Build history of the part. All positions in model axes, mm. A direction names the side the tool comes from. Give positions to 0.01 mm unless a question says otherwise; leave off trailing zeros. Write each loop counter-clockwise with the first axis right and the second up, starting at its lowest first coordinate (ties: lowest second). Pieces come first, ordered by that corner, then holes. Notation, with made-up numbers: (76.25, -11) -> (112.25, -11) arc R19 cw to (112.25, 0) -> close; hole circle Ø6 at (18, 19). An arc over 180 degrees is marked (long way). Write item = value, one per line. Start each with the question number.
Q1. Mould opens along X. For faces 1 (the face through (0, 28, 0)), 2 (the face through (-56, 1, 0)), 3 (the face through (-1, 1, 13.5)) say: pulls with the +X half, pulls with the -X half, needs draft (parallel to the pull), parting line crosses it, or undercut.
Q2. Saw through at D-D, the plane x = -32. List the corners of the cut face in (y, z).
Q3. Tool access for faces 4 (the face through (-47, 4, 0)), 5 (the face through (36.3, 4.6, 0.8)), 6 (the face through (47, 6.25, -1)), 7 (the face through (1, 1, -13.5)): list every direction of +Z, -Z, +X, -X, +Y, -Y with a clear straight run to the whole face (end or side of a thin tool).
Q4. Saw through at B-B, the plane x = 0. List the corners of the cut face in (y, z), then the cut area to 3 significant figures.
Q5. Saw through at A-A, the plane y = 25.5. List the corners of the cut face in (x, z).
Q6. Drop flat-ended pins along their axis: P1, Ø2.5, axis at x = 43, z = 2, coming from the +Y side; P2, Ø8, axis at x = -1, y = 17.5, coming from the -Z side; P3, Ø4, axis at x = 38, z = 3, coming from the +Y side; P4, Ø3, axis at x = 0, y = 25.5, coming from the +Z side. Give the stop position or say it passes through.
Q7. Wall check: line 1 (Y direction, x = 0, z = 1); line 2 (X direction, y = 2, z = 0); line 3 (X direction, y = 4.65, z = 0). Give the ranges that are in metal, low to high.
from build123d import *

# Parameters (mm, degrees)
BOSS_EXTRUDE1_DEPTH = 3
SKETCH7_R           = 5.75
BOSS_EXTRUDE5_DEPTH = 1
SKETCH2_R           = 3.75
CUT_EXTRUDE1_DEPTH  = 2.5
SKETCH3_R           = 6.25
BOSS_EXTRUDE3_DEPTH = 3.25
SKETCH4_R           = 4.25
CUT_EXTRUDE2_DEPTH  = 2.5
BOSS_EXTRUDE4_DEPTH = 27.5
SKETCH6_R           = 2.5
CUT_EXTRUDE3_DEPTH  = 67.327313378
FILLET1_R           = 0.5


with BuildPart() as part:
    # Sketch1 → Boss-Extrude1 (new body)
    with BuildSketch(Plane(origin=(0, 0, 0), x_dir=(1, 0, 0), z_dir=(0, 1, 0))):
        with BuildLine():
            Line((-42.5, -13.5), (42.5, -13.5))
            ThreePointArc((42.5, -13.5), (56, 0), (42.5, 13.5))
            Line((42.5, 13.5), (-42.5, 13.5))
            ThreePointArc((-42.5, 13.5), (-56, 0), (-42.5, -13.5))
        make_face()
    extrude(amount=BOSS_EXTRUDE1_DEPTH)

    # Sketch7 → Boss-Extrude5 (add)
    with BuildSketch(Plane(origin=(0, 3, 0), x_dir=(1, 0, 0), z_dir=(0, 1, 0))):
        with Locations(Location((-42.5, 0, 0), (0, 0, 270))):
            Circle(SKETCH7_R)
    extrude(amount=BOSS_EXTRUDE5_DEPTH)

    # Sketch2 → Cut-Extrude1 (cut)
    with BuildSketch(Plane(origin=(0, 4, 0), x_dir=(1, 0, 0), z_dir=(0, 1, 0))):
        with Locations(Location((-42.5, 0, 0), (0, 0, 270))):
            Circle(SKETCH2_R)
    extrude(amount=-CUT_EXTRUDE1_DEPTH, mode=Mode.SUBTRACT)

    # Sketch3 → Boss-Extrude3 (add)
    with BuildSketch(Plane(origin=(0, 3, 0), x_dir=(1, 0, 0), z_dir=(0, 1, 0))):
        with Locations(Location((42.5, 0, 0), (0, 0, 90))):
            Circle(SKETCH3_R)
    extrude(amount=BOSS_EXTRUDE3_DEPTH)

    # Sketch4 → Cut-Extrude2 (cut)
    with BuildSketch(Plane(origin=(0, 6.25, 0), x_dir=(1, 0, 0), z_dir=(0, 1, 0))):
        with Locations(Location((42.5, 0, 0), (0, 0, 270))):
            Circle(SKETCH4_R)
    extrude(amount=-CUT_EXTRUDE2_DEPTH, mode=Mode.SUBTRACT)

    # Sketch5 → Boss-Extrude4 (add)
    with BuildSketch(Plane(origin=(0, 3, 0), x_dir=(1, 0, 0), z_dir=(0, 1, 0))):
        with BuildLine():
            Line((-13.75, 4.75), (13.75, 4.75))
            ThreePointArc((13.75, 4.75), (18.5, 0), (13.75, -4.75))
            Line((13.75, -4.75), (-13.75, -4.75))
            ThreePointArc((-13.75, -4.75), (-18.5, 0), (-13.75, 4.75))
        make_face()
    extrude(amount=BOSS_EXTRUDE4_DEPTH)

    # Sketch6 → Cut-Extrude3 (cut, through all)
    with BuildSketch(Plane(origin=(0, 0, -4.75), x_dir=(-1, 0, 0), z_dir=(0, 0, -1))):
        with Locations((0, 25.5)):
            Circle(SKETCH6_R)
    extrude(amount=-CUT_EXTRUDE3_DEPTH, mode=Mode.SUBTRACT)

    # Fillet1
    fillet1_edges = [part.edges().sort_by_distance(p)[0] for p in [
        (-42.5, 3, -5.75),
        (-42.5, 4, -5.75),
        (-42.5, 4, -3.75),
    ]]
    fillet(fillet1_edges, radius=FILLET1_R - 0.0001)  # a hair under: the kernel refuses the full size


solid = part.part
Report:
q1.face_1 = undercut
q1.face_2 = pulls with the -X half
q1.face_3 = needs draft
q2.outline = (0, -13.5) -> (3, -13.5) -> (3, 13.5) -> (0, 13.5) -> close
q3.face_4 = +Z, -Z, -X, +Y
q3.face_5 = +Y
q3.face_6 = +Z, -Z, +X, +Y
q3.face_7 = -Z, +X, -X, +Y, -Y
q4.outline = (0, -13.5) -> (3, -13.5) -> (3, -4.75) -> (23, -4.75) -> (23, 4.75) -> (3, 4.75) -> (3, 13.5) -> (0, 13.5) -> close; (28, -4.75) -> (30.5, -4.75) -> (30.5, 4.75) -> (28, 4.75) -> close
q4.area = 295 mm2
q5.outline = (-13.75, -4.75) -> (-2.5, -4.75) -> (-2.5, 4.75) -> (-13.75, 4.75) arc R4.75 ccw to start; (2.5, -4.75) -> (13.75, -4.75) arc R4.75 ccw to (13.75, 4.75) -> (2.5, 4.75) -> close
q6.P1 = 3.75
q6.P2 = -4.75
q6.P3 = 6.25
q6.P4 = through
q7.line_1 = 0 to 23, 28 to 30.5
q7.line_2 = -56 to -46.25, -38.75 to 56
q7.line_3 = -18.5 to 18.5, 36.25 to 38.25, 46.75 to 48.75
